For this review, take the finished solid that the model builds, in its own axes (mm). A direction names the side the tool comes from. Give positions to 0.01 mm unless a question says otherwise; leave off trailing zeros. Loops run counter-clockwise (first coordinate to the right, second up) from the corner with the lowest first, then second, coordinate; pieces in that order, holes last.
```python
from build123d import *

# Parameters (mm, degrees)
CROQUIS1_W              = 100
CROQUIS1_H              = 100
SALIENTE_EXTRUIR1_DEPTH = 50
CROQUIS2_W              = 50
CROQUIS2_H              = 50
SALIENTE_EXTRUIR3_DEPTH = 50
SALIENTE_EXTRUIR4_DEPTH = 50


with BuildPart() as part:
    # Croquis1 → Saliente-Extruir1 (new body)
    with BuildSketch(Plane(origin=(0, 0, 0), x_dir=(1, 0, 0), z_dir=(0, 1, 0))):
        with Locations((9.571472252, 22.737819026)):
            Rectangle(CROQUIS1_W, CROQUIS1_H)
    extrude(amount=SALIENTE_EXTRUIR1_DEPTH)

    # Croquis2 → Saliente-Extruir3 (add)
    with BuildSketch(Plane(origin=(0, 50, 0), x_dir=(1, 0, 0), z_dir=(0, 1, 0))):
        with Locations((-15.428527748, 47.737819026)):
            Rectangle(CROQUIS2_W, CROQUIS2_H)
    extrude(amount=SALIENTE_EXTRUIR3_DEPTH)

    # Croquis3 → Saliente-Extruir4 (add)
    with BuildSketch(Plane(origin=(59.571472252, 0, 0), x_dir=(0, 0, -1), z_dir=(1, 0, 0))):
        Polygon((22.737819026, 50), (72.737819026, 100), (72.737819026, 50), align=None)
    extrude(amount=-SALIENTE_EXTRUIR4_DEPTH)


solid = part.part
```
Q1. Consider section C-C on y = 63. Give the boundary of the cut face in (x, z).
Answers:
outline: (-40.43, -72.74) - (59.57, -72.74) - (59.57, -35.74) - (9.57, -35.74) - (9.57, -22.74) - (-40.43, -22.74) - close
Q2. Consider section A-A on x = 13. Give the boundary of the cut face in (y, z), plus the area to 3 significant figures.
Answers:
outline: (0, -72.74) - (100, -72.74) - (50, -22.74) - (50, 27.26) - (0, 27.26) - close
area: 6,250 mm2
Q3. Consider section D-D on z = -4.5. Give the boundary of the cut face in (x, y), plus the area to 3 significant figures.
Answers:
outline: (-40.43, 0) - (59.57, 0) - (59.57, 50) - (-40.43, 50) - close
area: 5,000 mm2
Q4. Consider section B-B on z = -61. Give the boundary of the cut face in (x, y), plus the area to 3 significant figures.
Answers:
outline: (-40.43, 0) - (59.57, 0) - (59.57, 88.26) - (9.57, 88.26) - (9.57, 100) - (-40.43, 100) - close
area: 9,410 mm2
Q5. For probe 1 along X at (y, z) = (70.5, -37); probe 2 along Z at (x, y) = (-20, 62.5); probe 3 along Y at (x, z) = (-27, 5.5), list the stretches that pass through material, from the lowest coordinate up.
Answers:
probe 1: x = -40.43 to 9.57
probe 2: z = -72.74 to -22.74
probe 3: y = 0 to 50
Q6. Machinability: for faces 1 (the flat face through (-16, 75, -22.738)), 2 (the flat face through (34.92, 74.65, -47.39)), 3 (the flat face through (10, 51, -72.738)), which of the approach directions +Z, -Z, +X, -X, +Y, -Y give a long, thin tool a straight path to every point of the face, cutting with its end or side? Answer none if there is none.
Answers:
face 1: +Z, +X, -X, +Y
face 2: +Z, +X, +Y
face 3: -Z, +X, -X, +Y, -Y
